Geometry check sheet. Reference: drawing and pictorial views, mm from the part's lowest x, y, z. A direction names the side the tool comes from. Give positions to 0.01 mm unless a question says otherwise; leave off trailing zeros. Loops run counter-clockwise (first coordinate to the right, second up) from the corner with the lowest first, then second, coordinate; pieces in that order, holes last. Notation, with made-up numbers: (13, 85.25) -> (46, 85.25) arc R17 ccw to (46, 110.25) -> close; hole circle Ø11 at (-10.5, 79.25). An arc over 180 degrees is marked (long way). One line per item, written item: value. Start each with the question number.
(1) Tool access check on the marked faces 1, 2, 3 and 4. Record the directions out of +Z, -Z, +X, -X, +Y, -Y that give a thin tool (end or side, any length) a straight path to the whole face; none if there is none.
(2) Sectioned sample at D-D, the plane x = 28. Record the cut outline in (y, z).
(3) Sectioned sample at B-B, the plane y = 7.5. Record the cut outline in (x, z), then the cut area to 3 significant figures.
(4) Scan lines: line 1 along Y through (x, z) = (30, 18.1); line 2 along X through (y, z) = (5.75, 17.7); line 3 along Z through (x, y) = (19.5, 2.5). Record each from-to range of solid material in increasing order. Write a range as from..to.
(5) Sectioned sample at C-C, the plane z = 14.75. Record the cut outline in (x, y).
(6) Gauge pin test, flat ends, axial feed: pin 1 Ø2 at (y, z) = (5.5, 9) entering from +X; pin 2 Ø6 at (y, z) = (5.5, 13) entering from -X; pin 3 Ø3.5 at (x, y) = (30, 5.75) entering from +Z. Record the tip position at first contact, or that the pin passes through.
(7) Sectioned sample at A-A, the plane x = 2. Record the cut outline in (y, z), then the cut area to 3 significant figures.
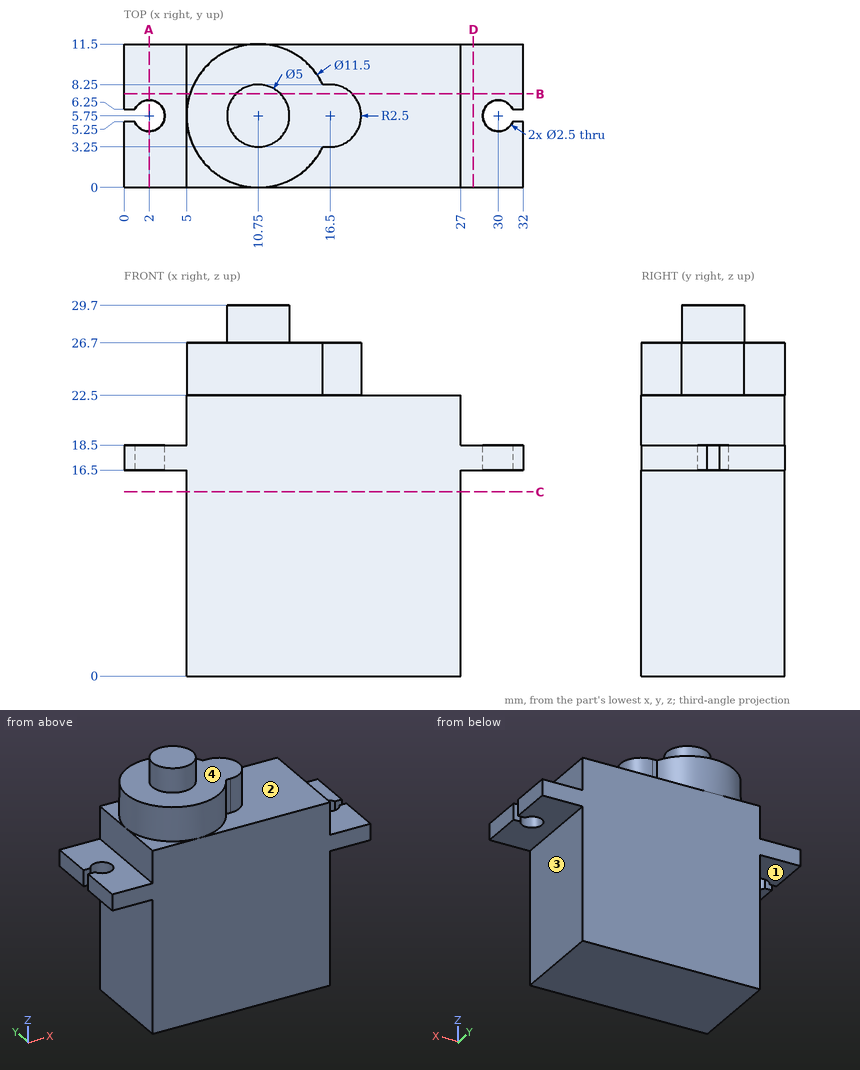
Calculated:
1. face 1: -Z, -X, +Y, -Y
1. face 2: +Z, +X
1. face 3: -Z, +X, +Y, -Y
1. face 4: +Z
2. outline: (0, 16.5) -> (11.5, 16.5) -> (11.5, 18.5) -> (0, 18.5) -> close
3. outline: (0, 16.5) -> (5, 16.5) -> (5, 0) -> (27, 0) -> (27, 16.5) -> (32, 16.5) -> (32, 18.5) -> (27, 18.5) -> (27, 22.5) -> (18.29, 22.5) -> (18.29, 26.7) -> (12.54, 26.7) -> (12.54, 29.7) -> (8.96, 29.7) -> (8.96, 26.7) -> (5.27, 26.7) -> (5.27, 22.5) -> (5, 22.5) -> (5, 18.5) -> (0, 18.5) -> close
3. area: 580 mm2
4. line 1: y = 0..4.5, 7..11.5
4. line 2: x = 3.25..28.75
4. line 3: z = 0..22.5
5. outline: (5, 0) -> (27, 0) -> (27, 11.5) -> (5, 11.5) -> close
6. pin 1: stops at x = 27
6. pin 2: stops at x = 5
6. pin 3: stops at z = 18.5
7. outline: (0, 16.5) -> (4.5, 16.5) -> (4.5, 18.5) -> (0, 18.5) -> close; (7, 16.5) -> (11.5, 16.5) -> (11.5, 18.5) -> (7, 18.5) -> close
7. area: 18.0 mm2
